from build123d import *

# Parameters (mm, degrees)
BOSS_EXTRUDE1_DEPTH = 4.5


with BuildPart() as part:
    # Sketch1 → Boss-Extrude1 (new body)
    with BuildSketch(Plane(origin=(0, 0, 0), x_dir=(1, 0, 0), z_dir=(0, 1, 0))):
        with BuildLine():
            Line((-10, 0), (-10, 15))
            Line((-10, 15), (10, 15))
            Line((10, 15), (10, 0))
            Line((10, 0), (6, 0))
            Line((6, 0), (6, -11.5))
            ThreePointArc((6, -11.5), (5.414213562, -12.914213562), (4, -13.5))
            Line((4, -13.5), (-4, -13.5))
            ThreePointArc((-4, -13.5), (-5.414213562, -12.914213562), (-6, -11.5))
            Line((-6, -11.5), (-6, 0))
            Line((-6, 0), (-10, 0))
        make_face()
        with BuildLine():
            Line((2.25, 0), (2.25, -8.133974596))
            ThreePointArc((2.25, -8.133974596), (2.316987298, -8.383974596), (2.5, -8.566987298))
            ThreePointArc((2.5, -8.566987298), (2.732962913, -9.129409523), (2.25, -9.5))
            Line((2.25, -9.5), (-2.25, -9.5))
            ThreePointArc((-2.25, -9.5), (-2.732962913, -9.129409523), (-2.5, -8.566987298))
            ThreePointArc((-2.5, -8.566987298), (-2.316987298, -8.383974596), (-2.25, -8.133974596))
            Line((-2.25, -8.133974596), (-2.25, 0))
            ThreePointArc((-2.25, 0), (0, 2.25), (2.25, 0))
        make_face(mode=Mode.SUBTRACT)
    extrude(amount=BOSS_EXTRUDE1_DEPTH)


solid = part.part
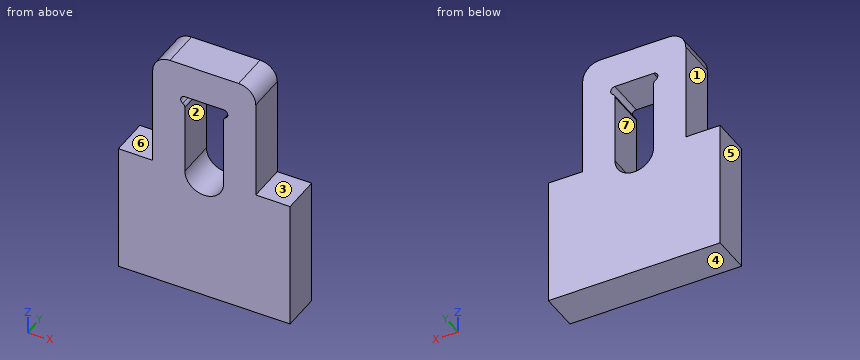
Check sheet for the modelled part. Datum: model origin and axes. Units: mm. Face numbers are marked on the shaded views. A direction names the side the tool comes from. Give positions to 0.01 mm unless a question says otherwise; leave off trailing zeros. Order: outer loops, then holes, each group sorted by start corner. A loop starts at its lowest first (then second) coordinate and runs counter-clockwise, first axis right, second up. Notation, with made-up numbers: M -34,-29 L -9,-29 A25 ccw -9,3 Z; hole C 76.5,84.5 d5. An arc over 180 degrees is marked long. Answer as CSV lines item,"result". Start each with the question number.
Item 1: Tool access check on the marked faces 1, 2 and 3. Record the directions out of +Z, -Z, +X, -X, +Y, -Y that give a thin tool (end or side, any length) a straight path to the whole face; none if there is none.
Item 2: Thickness scan on line 1 (X direction, y = 0.35, z = 7.25); line 2 (X direction, y = 4.35, z = 9); line 3 (Z direction, x = 0.5, y = 3.8). Record the ranges inside material, lowest first. Write a range as [from, to].
Item 3: Mould release check, pull along Z, two halves, no side actions. Record for the marked faces 4, 5, 6 and 7: +Z half, -Z half, draft (parallel to the pull), parting line (faces both ways), or undercut.
Item 4: Cross-section at D-D on x = -8.5. Enter the section's corners in (y, z).
Item 5: Cross-section at B-B on z = 7.5. Enter the section's corners in (x, y), plus the area to 4 significant figures.
Item 6: Gauge pin test, flat ends, axial feed: P1, Ø1.2, axis at x = -8.5, y = 3, coming from the +Z side; P2, Ø2, axis at y = 3, z = 3.5, coming from the +X side; P3, Ø10, axis at x = 1.5, z = 7, coming from the +Y side. Record the tip position at first contact, or that the pin passes through.
Item 7: Cross-section at C-C on y = 2.75. Enter the section's corners in (x, z), plus the area to 3 significant figures.
Item 8: Cross-section at A-A on x = 0. Enter the section's corners in (y, z), plus the area to 3 significant figures.
Established:
1,face 1,"+Z, -X, +Y, -Y"
1,face 2,"+Y, -Y"
1,face 3,"+Z, +X, +Y, -Y"
2,line 1,"x = [-6, -2.25], [2.25, 6]"
2,line 2,"x = [-6, -2.75], [2.75, 6]"
2,line 3,"z = [-15, -2.19], [9.5, 13.5]"
3,face 4,"-Z half"
3,face 5,"draft"
3,face 6,"+Z half"
3,face 7,"undercut"
4,outline,"M 0,-15 L 4.5,-15 L 4.5,0 L 0,0 Z"
5,outline,"M -6,0 L -2.25,0 L -2.25,4.5 L -6,4.5 Z; M 2.25,0 L 6,0 L 6,4.5 L 2.25,4.5 Z"
5,area,"33.75 mm^2"
6,P1,"stops at z = 0"
6,P2,"stops at x = 6"
6,P3,"stops at y = 4.5"
7,outline,"M -10,-15 L 10,-15 L 10,0 L 6,0 L 6,11.5 A2 ccw 4,13.5 L -4,13.5 A2 ccw -6,11.5 L -6,0 L -10,0 Z; hole M -2.5,8.57 A0.5 cw -2.25,8.13 L -2.25,0 A2.25 ccw 2.25,0 L 2.25,8.13 A0.5 cw 2.5,8.57 A0.5 ccw 2.25,9.5 L -2.25,9.5 A0.5 ccw Z"
7,area,"409 mm^2"
8,outline,"M 0,-15 L 4.5,-15 L 4.5,-2.25 L 0,-2.25 Z; M 0,9.5 L 4.5,9.5 L 4.5,13.5 L 0,13.5 Z"
8,area,"75.4 mm^2"
